from build123d import *

# Parameters (mm, degrees)
BOSS_EXTRUDE1_DEPTH = 7.95
SKETCH2_R           = 2.4
BOSS_EXTRUDE2_DEPTH = 1.8
LPATTERN1_COUNT     = 4
LPATTERN1_PITCH     = 8
SHELL3_T            = -1.2
CUT_EXTRUDE1_START  = -1.2
SKETCH3_W           = 15.9
SKETCH3_H           = 5.55
CUT_EXTRUDE1_DEPTH  = 29.546176225


with BuildPart() as part:
    # Sketch1 → Boss-Extrude1 (new body)
    with BuildSketch(Plane.XY):
        with BuildLine():
            Line((-7.95, 0), (-15.9, 0))
            Line((-15.9, 0), (-15.9, 23.85))
            Line((-15.9, 23.85), (15.9, 23.85))
            Line((15.9, 23.85), (15.9, 0))
            Line((15.9, 0), (7.95, 0))
            Line((7.95, 0), (7.95, 15.9))
            ThreePointArc((7.95, 15.9), (0, 20.65), (-7.95, 15.9))
            Line((-7.95, 15.9), (-7.95, 0))
        make_face()
    extrude(amount=-BOSS_EXTRUDE1_DEPTH)

    # Sketch2 → Boss-Extrude2 (add)
    with BuildSketch(Plane(origin=(0, 23.85, 0), x_dir=(1, 0, 0), z_dir=(0, 1, 0))):
        with Locations(Location((-12, 4.05, 0), (0, 0, 270))):
            Circle(SKETCH2_R)
    boss_extrude2 = extrude(amount=BOSS_EXTRUDE2_DEPTH)

    # LPattern1: Boss-Extrude2 ×4
    with Locations(*[(i * LPATTERN1_PITCH, 0, 0) for i in range(1, LPATTERN1_COUNT)]):
        add(boss_extrude2)

    # Shell3
    shell3_openings = [part.faces().sort_by_distance(p)[0] for p in [
        (-11.925, 0, -3.975),
        (11.925, 0, -3.975),
    ]]
    offset(amount=SHELL3_T, openings=shell3_openings, kind=Kind.INTERSECTION)

    # Sketch3 → Cut-Extrude1 (cut, through all)
    with BuildSketch(Plane(origin=(0, 23.85, 0), x_dir=(1, 0, 0), z_dir=(0, 1, 0)).offset(CUT_EXTRUDE1_START)):
        with Locations((0, 3.975)):
            Rectangle(SKETCH3_W, SKETCH3_H)
    extrude(amount=-CUT_EXTRUDE1_DEPTH, mode=Mode.SUBTRACT)


solid = part.part
Verification items for the finished model (mm, model axes). A direction names the side the tool comes from. Coordinates: 2 decimals unless noted, no trailing zeros. Loops run counter-clockwise (first coordinate to the right, second up) from the corner with the lowest first, then second, coordinate; pieces in that order, holes last. Notation, with made-up numbers: (-33, 40) -> (-28, 40) arc R14 cw to (-28, 49) -> close; hole circle Ø4 at (77, 83.5). An arc over 180 degrees is marked (long way). Write each question's results on one line, items separated by ' | '.
Item 1: Section check D-D, the plane y = 20.25. Enter the section's corners in (x, z), plus the area to 3 significant figures.
Found:
outline: (-15.9, -7.95) -> (-2.66, -7.95) -> (-2.66, -6.75) -> (-14.7, -6.75) -> (-14.7, -1.2) -> (-2.66, -1.2) -> (-2.66, 0) -> (-15.9, 0) -> close; (2.66, -7.95) -> (15.9, -7.95) -> (15.9, 0) -> (2.66, 0) -> (2.66, -1.2) -> (14.7, -1.2) -> (14.7, -6.75) -> (2.66, -6.75) -> close | area: 76.9 mm2
Item 2: Section check C-C, the plane z = -2.5. Count the separate pieces of the cut face and the enclosed holes in it, plus the area to 3 significant figures.
Found:
separate pieces: 3 | enclosed holes: 0 | area: 160 mm2
Item 3: Section check A-A, the plane y = 7.5. Enter the section's corners in (x, z), plus the area to 3 significant figures.
Found:
outline: (-15.9, -7.95) -> (-7.95, -7.95) -> (-7.95, 0) -> (-15.9, 0) -> close; (7.95, -7.95) -> (15.9, -7.95) -> (15.9, 0) -> (7.95, 0) -> close; hole (-14.7, -6.75) -> (-9.15, -6.75) -> (-9.15, -1.2) -> (-14.7, -1.2) -> close; hole (9.15, -6.75) -> (14.7, -6.75) -> (14.7, -1.2) -> (9.15, -1.2) -> close | area: 64.8 mm2
Item 4: Mould release check, pull along Z, two halves, no side actions. Record for faces 1 (the face through (-5.17, 23.54, -4.31)), 2 (the face through (12, 25.65, -4)), 3 (the face through (4, 20, -7.95)): +Z half, -Z half, draft (parallel to the pull), parting line (faces both ways), or undercut.
Found:
face 1: undercut | face 2: draft | face 3: -Z half
Item 5: Section check B-B, the plane x = 0. Enter the section's corners in (y, z).
Found:
outline: (20.65, -7.95) -> (23.85, -7.95) -> (23.85, 0) -> (20.65, 0) -> (20.65, -1.2) -> (22.65, -1.2) -> (22.65, -6.75) -> (20.65, -6.75) -> close
Item 6: Material ranges on L1, parallel to X at y = 9.5, z = -2.25; L2, parallel to X at y = 23.1, z = -4.05; L3, parallel to Z at x = -12, y = 23.25, recorded low to high.
Found:
L1: x = -15.9 to -14.7, -9.15 to -7.95, 7.95 to 9.15, 14.7 to 15.9 | L2: x = -15.9 to -13.2, -10.8 to -5.2, -2.8 to 2.8, 5.2 to 10.8, 13.2 to 15.9 | L3: z = -7.95 to -5.25, -2.85 to 0
Item 7: Tool access check on faces 4 (the face through (8.61, 17.14, -3.94)), 5 (the face through (0.14, 20.65, -7.34)), 6 (the face through (-12, 25.65, -4)), 7 (the face through (0, 23.85, -4)), 8 (the face through (-12, 24.45, -4)). Record the directions out of +Z, -Z, +X, -X, +Y, -Y that give a thin tool (end or side, any length) a straight path to the whole face; none if there is none.
Found:
face 4: none | face 5: +Z, -Z, -Y | face 6: +Z, -Z, +X, -X, +Y | face 7: +Y | face 8: -Y
Item 8: Gauge pin test, flat ends, axial feed: pin 1 (1 mm diameter, centred on x = 4, z = -6.5, fed in from -Y); pin 2 (2.5 mm diameter, centred on x = 11.5, z = -4.5, fed in from -Y); pin 3 (0.7 mm diameter, centred on x = -3.5, z = -4.5, fed in from -Y). Record the tip position at first contact, or that the pin passes through.
Found:
pin 1: stops at y = 19.49 | pin 2: stops at y = 22.65 | pin 3: stops at y = 24.45
